from build123d import *

# Parameters (mm, degrees)
ESTRUSIONE_ESTRUSIONE1_DEPTH = 140
FORO_6_5_6_5_1_D             = 6.5
FORO_6_5_6_5_2_D             = 6.5
FORO_6_5_6_5_2_DEPTH         = 5
FORO_6_5_6_5_2_TIP           = 1.952797012
TAGLIO_ESTRUSIONE3_REACH     = 158.844
SCHIZZO10_R                  = 1.75
SCHIZZO10_R_2                = 7
TAGLIO_ESTRUSIONE4_REACH     = 158.844
SCHIZZO11_R                  = 1.75
TAGLIO_ESTRUSIONE6_REACH     = 158.844
SMUSSO1_SIZE                 = 3


with BuildPart() as part:
    # Schizzo1 → Estrusione-Estrusione1 (new body)
    with BuildSketch(Plane.XY):
        Polygon((0, 0), (0, 50), (5, 50), (5, 5), (50, 5), (50, 0), align=None)
    extrude(amount=ESTRUSIONE_ESTRUSIONE1_DEPTH)

    # Foro Ø6.5 (6.5)-1 (through all)
    with Locations(Plane(origin=(0, 0, 0), x_dir=(-1, 0, 0), z_dir=(0, -1, 0))):
        with Locations((-17, -132), (-42, -132)):
            foro_6_5_6_5_1 = Hole(FORO_6_5_6_5_1_D / 2)

    # Foro Ø6.5 (6.5)-2
    with Locations(Plane.ZY):
        with Locations((132, 42), (132, 17)):
            Hole(FORO_6_5_6_5_2_D / 2, depth=FORO_6_5_6_5_2_DEPTH)
            with Locations((0, 0, -(FORO_6_5_6_5_2_DEPTH + FORO_6_5_6_5_2_TIP / 2))):  # 118° drill point
                Cone(0, FORO_6_5_6_5_2_D / 2, FORO_6_5_6_5_2_TIP, mode=Mode.SUBTRACT)

    # Specchia1: Foro Ø6.5 (6.5)-1 across plane
    add(foro_6_5_6_5_1.mirror(Plane.XY.offset(70)), mode=Mode.SUBTRACT)

    # Schizzo10 → Taglio-Estrusione3 (cut, up to next)
    with BuildSketch(Plane.ZY, mode=Mode.PRIVATE) as taglio_estrusione3_sk1:
        with Locations((70, 40)):
            Circle(SCHIZZO10_R)
    taglio_estrusione3_tool1 = extrude(taglio_estrusione3_sk1.sketch, amount=-TAGLIO_ESTRUSIONE3_REACH, mode=Mode.PRIVATE) & part.part
    # Schizzo10 → Taglio-Estrusione3 (cut, up to next)
    with BuildSketch(Plane.ZY, mode=Mode.PRIVATE) as taglio_estrusione3_sk2:
        with Locations((90, 40)):
            Circle(SCHIZZO10_R)
    taglio_estrusione3_tool2 = extrude(taglio_estrusione3_sk2.sketch, amount=-TAGLIO_ESTRUSIONE3_REACH, mode=Mode.PRIVATE) & part.part
    # Schizzo10 → Taglio-Estrusione3 (cut, up to next)
    with BuildSketch(Plane.ZY, mode=Mode.PRIVATE) as taglio_estrusione3_sk3:
        with Locations((90, 20)):
            Circle(SCHIZZO10_R)
    taglio_estrusione3_tool3 = extrude(taglio_estrusione3_sk3.sketch, amount=-TAGLIO_ESTRUSIONE3_REACH, mode=Mode.PRIVATE) & part.part
    # Schizzo10 → Taglio-Estrusione3 (cut, up to next)
    with BuildSketch(Plane.ZY, mode=Mode.PRIVATE) as taglio_estrusione3_sk4:
        with Locations((70, 20)):
            Circle(SCHIZZO10_R)
    taglio_estrusione3_tool4 = extrude(taglio_estrusione3_sk4.sketch, amount=-TAGLIO_ESTRUSIONE3_REACH, mode=Mode.PRIVATE) & part.part
    # Schizzo10 → Taglio-Estrusione3 (cut, up to next)
    with BuildSketch(Plane.ZY, mode=Mode.PRIVATE) as taglio_estrusione3_sk5:
        with Locations((80, 30)):
            Circle(SCHIZZO10_R_2)
    taglio_estrusione3_tool5 = extrude(taglio_estrusione3_sk5.sketch, amount=-TAGLIO_ESTRUSIONE3_REACH, mode=Mode.PRIVATE) & part.part
    add(taglio_estrusione3_tool1.solids().sort_by_distance((0, 40, 70))[0], mode=Mode.SUBTRACT)
    add(taglio_estrusione3_tool2.solids().sort_by_distance((0, 40, 90))[0], mode=Mode.SUBTRACT)
    add(taglio_estrusione3_tool3.solids().sort_by_distance((0, 20, 90))[0], mode=Mode.SUBTRACT)
    add(taglio_estrusione3_tool4.solids().sort_by_distance((0, 20, 70))[0], mode=Mode.SUBTRACT)
    add(taglio_estrusione3_tool5.solids().sort_by_distance((0, 30, 80))[0], mode=Mode.SUBTRACT)

    # Schizzo11 → Taglio-Estrusione4 (cut, up to next)
    with BuildSketch(Plane.XZ, mode=Mode.PRIVATE) as taglio_estrusione4_sk1:
        with Locations((20, 90)):
            Circle(SCHIZZO11_R)
    taglio_estrusione4_tool1 = extrude(taglio_estrusione4_sk1.sketch, amount=-TAGLIO_ESTRUSIONE4_REACH, mode=Mode.PRIVATE) & part.part
    # Schizzo11 → Taglio-Estrusione4 (cut, up to next)
    with BuildSketch(Plane.XZ, mode=Mode.PRIVATE) as taglio_estrusione4_sk2:
        with Locations((20, 110)):
            Circle(SCHIZZO11_R)
    taglio_estrusione4_tool2 = extrude(taglio_estrusione4_sk2.sketch, amount=-TAGLIO_ESTRUSIONE4_REACH, mode=Mode.PRIVATE) & part.part
    # Schizzo11 → Taglio-Estrusione4 (cut, up to next)
    with BuildSketch(Plane.XZ, mode=Mode.PRIVATE) as taglio_estrusione4_sk3:
        with Locations((40, 110)):
            Circle(SCHIZZO11_R)
    taglio_estrusione4_tool3 = extrude(taglio_estrusione4_sk3.sketch, amount=-TAGLIO_ESTRUSIONE4_REACH, mode=Mode.PRIVATE) & part.part
    # Schizzo11 → Taglio-Estrusione4 (cut, up to next)
    with BuildSketch(Plane.XZ, mode=Mode.PRIVATE) as taglio_estrusione4_sk4:
        with Locations((40, 90)):
            Circle(SCHIZZO11_R)
    taglio_estrusione4_tool4 = extrude(taglio_estrusione4_sk4.sketch, amount=-TAGLIO_ESTRUSIONE4_REACH, mode=Mode.PRIVATE) & part.part
    add(taglio_estrusione4_tool1.solids().sort_by_distance((20, 0, 90))[0], mode=Mode.SUBTRACT)
    add(taglio_estrusione4_tool2.solids().sort_by_distance((20, 0, 110))[0], mode=Mode.SUBTRACT)
    add(taglio_estrusione4_tool3.solids().sort_by_distance((40, 0, 110))[0], mode=Mode.SUBTRACT)
    add(taglio_estrusione4_tool4.solids().sort_by_distance((40, 0, 90))[0], mode=Mode.SUBTRACT)

    # Schizzo13 → Taglio-Estrusione6 (cut, up to next)
    with BuildSketch(Plane.ZY, mode=Mode.PRIVATE) as taglio_estrusione6_sk1:
        with BuildLine():
            Line((15.443650814, 43.306349186), (23.443650814, 43.306349186))
            ThreePointArc((23.443650814, 43.306349186), (25.193650814, 41.556349186), (23.443650814, 39.806349186))
            Line((23.443650814, 39.806349186), (15.443650814, 39.806349186))
            ThreePointArc((15.443650814, 39.806349186), (13.693650814, 41.556349186), (15.443650814, 43.306349186))
        make_face()
    taglio_estrusione6_tool1 = extrude(taglio_estrusione6_sk1.sketch, amount=-TAGLIO_ESTRUSIONE6_REACH, mode=Mode.PRIVATE) & part.part
    # Schizzo13 → Taglio-Estrusione6 (cut, up to next)
    with BuildSketch(Plane.ZY, mode=Mode.PRIVATE) as taglio_estrusione6_sk2:
        with BuildLine():
            Line((15.443650814, 8.693650814), (23.443650814, 8.693650814))
            ThreePointArc((23.443650814, 8.693650814), (25.193650814, 10.443650814), (23.443650814, 12.193650814))
            Line((23.443650814, 12.193650814), (15.443650814, 12.193650814))
            ThreePointArc((15.443650814, 12.193650814), (13.693650814, 10.443650814), (15.443650814, 8.693650814))
        make_face()
    taglio_estrusione6_tool2 = extrude(taglio_estrusione6_sk2.sketch, amount=-TAGLIO_ESTRUSIONE6_REACH, mode=Mode.PRIVATE) & part.part
    # Schizzo13 → Taglio-Estrusione6 (cut, up to next)
    with BuildSketch(Plane.ZY, mode=Mode.PRIVATE) as taglio_estrusione6_sk3:
        with BuildLine():
            Line((54.556349186, 43.306349186), (46.556349186, 43.306349186))
            ThreePointArc((46.556349186, 43.306349186), (44.806349186, 41.556349186), (46.556349186, 39.806349186))
            Line((46.556349186, 39.806349186), (54.556349186, 39.806349186))
            ThreePointArc((54.556349186, 39.806349186), (56.306349186, 41.556349186), (54.556349186, 43.306349186))
        make_face()
    taglio_estrusione6_tool3 = extrude(taglio_estrusione6_sk3.sketch, amount=-TAGLIO_ESTRUSIONE6_REACH, mode=Mode.PRIVATE) & part.part
    # Schizzo13 → Taglio-Estrusione6 (cut, up to next)
    with BuildSketch(Plane.ZY, mode=Mode.PRIVATE) as taglio_estrusione6_sk4:
        with BuildLine():
            Line((54.556349186, 8.693650814), (46.556349186, 8.693650814))
            ThreePointArc((46.556349186, 8.693650814), (44.806349186, 10.443650814), (46.556349186, 12.193650814))
            Line((46.556349186, 12.193650814), (54.556349186, 12.193650814))
            ThreePointArc((54.556349186, 12.193650814), (56.306349186, 10.443650814), (54.556349186, 8.693650814))
        make_face()
    taglio_estrusione6_tool4 = extrude(taglio_estrusione6_sk4.sketch, amount=-TAGLIO_ESTRUSIONE6_REACH, mode=Mode.PRIVATE) & part.part
    # Schizzo13 → Taglio-Estrusione6 (cut, up to next)
    with BuildSketch(Plane.ZY, mode=Mode.PRIVATE) as taglio_estrusione6_sk5:
        with BuildLine():
            Line((40, 14.75), (30, 14.75))
            ThreePointArc((30, 14.75), (18.75, 26), (30, 37.25))
            Line((30, 37.25), (40, 37.25))
            ThreePointArc((40, 37.25), (51.25, 26), (40, 14.75))
        make_face()
    taglio_estrusione6_tool5 = extrude(taglio_estrusione6_sk5.sketch, amount=-TAGLIO_ESTRUSIONE6_REACH, mode=Mode.PRIVATE) & part.part
    add(taglio_estrusione6_tool1.solids().sort_by_distance((0, 41.556349, 19.443651))[0], mode=Mode.SUBTRACT)
    add(taglio_estrusione6_tool2.solids().sort_by_distance((0, 10.443651, 19.443651))[0], mode=Mode.SUBTRACT)
    add(taglio_estrusione6_tool3.solids().sort_by_distance((0, 41.556349, 50.556349))[0], mode=Mode.SUBTRACT)
    add(taglio_estrusione6_tool4.solids().sort_by_distance((0, 10.443651, 50.556349))[0], mode=Mode.SUBTRACT)
    add(taglio_estrusione6_tool5.solids().sort_by_distance((0, 26, 35))[0], mode=Mode.SUBTRACT)

    # Smusso1
    smusso1_edges = [part.edges().sort_by_distance(p)[0] for p in [
        (2.5, 50, 140),
        (2.5, 50, 0),
        (50, 2.5, 140),
        (50, 2.5, 0),
    ]]
    chamfer(smusso1_edges, length=SMUSSO1_SIZE)


solid = part.part
Build history of the part. All positions in model axes, mm. A direction names the side the tool comes from. Round coordinates to 2 decimals unless told otherwise and drop trailing zeros. Order: outer loops, then holes, each group sorted by start corner. A loop starts at its lowest first (then second) coordinate and runs counter-clockwise, first axis right, second up. Notation, with made-up numbers: M -23,37 L -9,37 A29 ccw -9,71 Z; hole C 46,54 d1. An arc over 180 degrees is marked long. Use CSV: the item, a comma, the result in double quotes. Start each with the question number.
(1) Drill centre lines: probe 1 along Z at (x, y) = (17, 1.3); probe 2 along X at (y, z) = (2, 90). Where is each one in solid material? Low to high.
(2) Flat gauge pin, fed straight in: P1, Ø5.5, axis at x = 40, z = 110, coming from the +Y side. Where does the tip first touch, or does it go through?
(3) Cut at D-D on x = 9.5. List the corners of the cut face in (y, z), then the cut area to 3 significant figures.
(4) Tool access for faces 1 (the face through (49, 3, 138)), 2 (the face through (2, 14.75, 35)), 3 (the face through (27, 5, 69)): list every direction of +Z, -Z, +X, -X, +Y, -Y with a clear straight run to the whole face (end or side of a thin tool).
(5) Cut at B-B on z = 8. List the corners of the cut face in (x, y).
(6) Cut at A-A on z = 80. List the corners of the cut face in (x, y), then the cut area to 3 significant figures.
(7) Mould opens along Y. For faces 4 (the face through (2, 49, 138)), 5 (the face through (40.9, 2.5, 111.5)), 6 (the face through (2.465, 25.753, 18.753)) say: +Y half, -Y half, draft (parallel to the pull), parting line (faces both ways), or undercut.
(8) Cut at C-C on y = 27. List the corners of the cut face in (x, z), then the cut area to 3 significant figures.
Findings:
1,probe 1,"z = 0 to 4.75, 11.25 to 128.75, 135.25 to 140"
1,probe 2,"x = 0 to 18.25, 21.75 to 38.25, 41.75 to 50"
2,P1,"stops at y = 5"
3,outline,"M 0,0 L 5,0 L 5,140 L 0,140 Z"
3,area,"700 mm^2"
4,face 1,"+Z, +X, +Y, -Y"
4,face 2,"+X, -X"
4,face 3,"+Z, -Z, +X, +Y"
5,outline,"M 0,0 L 13.75,0 L 13.75,5 L 5,5 L 5,50 L 0,50 Z; M 20.25,0 L 38.75,0 L 38.75,5 L 20.25,5 Z; M 45.25,0 L 50,0 L 50,5 L 45.25,5 Z"
6,outline,"M 0,0 L 50,0 L 50,5 L 5,5 L 5,23 L 0,23 Z; M 0,37 L 5,37 L 5,50 L 0,50 Z"
6,area,"405 mm^2"
7,face 4,"+Y half"
7,face 5,"draft"
7,face 6,"undercut"
8,outline,"M 0,0 L 5,0 L 5,18.79 L 0,18.79 Z; M 0,51.21 L 5,51.21 L 5,73.68 L 0,73.68 Z; M 0,86.32 L 5,86.32 L 5,140 L 0,140 Z"
8,area,"475 mm^2"
